Verification items for this drawing (mm, ordinates from the low corner). A direction names the side the tool comes from. Give positions to 0.01 mm unless a question says otherwise; leave off trailing zeros. Loops run counter-clockwise (first coordinate to the right, second up) from the corner with the lowest first, then second, coordinate; pieces in that order, holes last. Notation, with made-up numbers: M -3.75,80 L 17.25,80 A11 ccw 17.25,88 Z; hole C -6.75,12.5 d9. An arc over 180 degrees is marked long. Use a Markdown table: item, result.
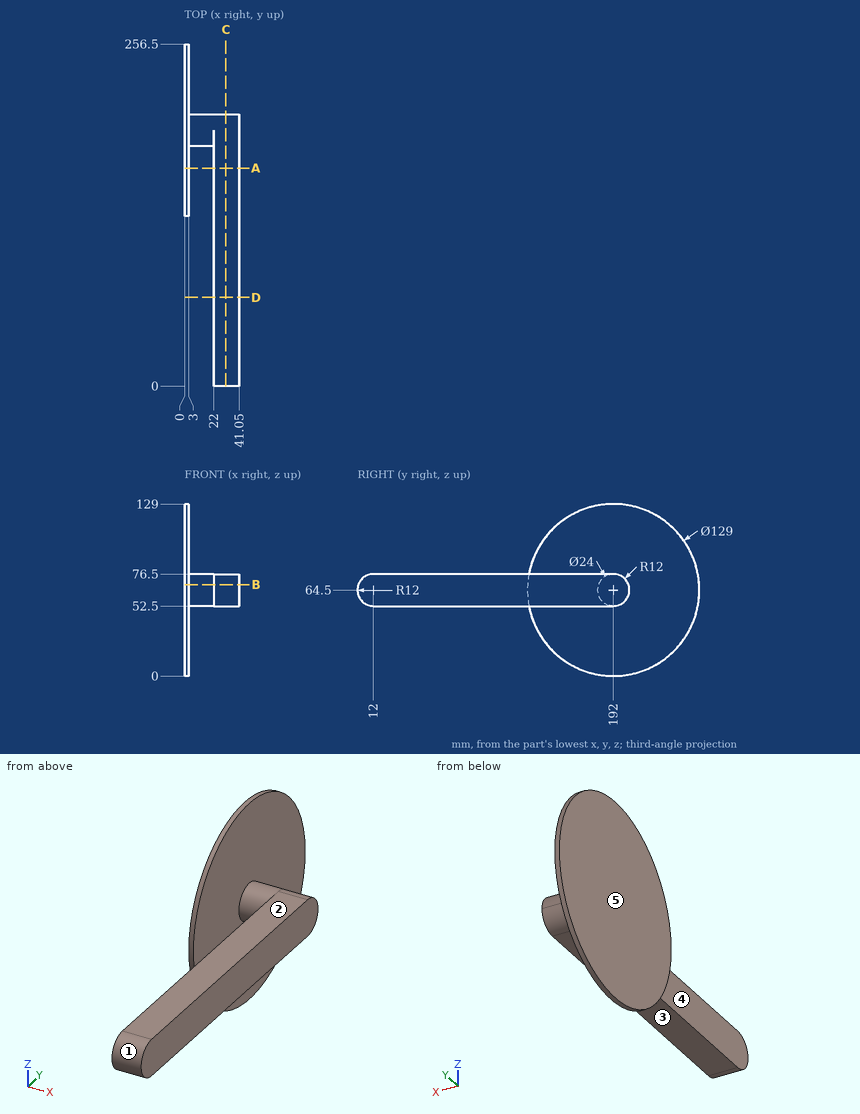
(1) Cross-section at B-B on z = 68.5. Record the cut outline in (x, y), then the cut area to 3 significant figures.
Results below:
| item | result |
|---|---|
| outline | M 0,127.62 L 3,127.62 L 3,180.69 L 22,180.69 L 22,0.69 L 41.05,0.69 L 41.05,203.31 L 3,203.31 L 3,256.38 L 0,256.38 Z |
| area | 4,680 mm^2 |
(2) Cross-section at A-A on y = 163.5. Record the cut outline in (x, z).
Results below:
| item | result |
|---|---|
| outline | M 0,6.64 L 3,6.64 L 3,122.36 L 0,122.36 Z; M 22,52.5 L 41.05,52.5 L 41.05,76.5 L 22,76.5 Z |
(3) Set-up check for the marked faces 1 and 2: record each of +Z, -Z, +X, -X, +Y, -Y from which the full face is reachable in a straight line by a thin tool's end or side.
Results below:
| item | result |
|---|---|
| face 1 | +X, -X, -Y |
| face 2 | +Z, +X, +Y, -Y |
(4) Gauge pin test, flat ends, axial feed: P1, Ø4, axis at x = 29, y = 111.5, coming from the +Z side; P2, Ø15, axis at x = 27, y = 59, coming from the -Z side; P3, Ø12, axis at x = 6.5, z = 14, coming from the -Y side. Record the tip position at first contact, or that the pin passes through.
Results below:
| item | result |
|---|---|
| P1 | z = 76.5 |
| P2 | z = 52.5 |
| P3 | y = 146.41 |
(5) Cross-section at C-C on x = 31. Record the cut outline in (y, z).
Results below:
| item | result |
|---|---|
| outline | M 12,52.5 L 192,52.5 A12 ccw 204,64.5 A12 ccw 192,76.5 L 12,76.5 A12 ccw Z |
(6) Draft check along X on the marked faces 3, 4 and 5. Enter one of: +X half, -X half, draft (parallel to the pull), parting line (faces both ways), or undercut.
Results below:
| item | result |
|---|---|
| face 3 | draft |
| face 4 | undercut |
| face 5 | -X half |
(7) Material ranges on line 1 (X direction, y = 178, z = 64); line 2 (Z direction, x = 29.5, y = 53); line 3 (X direction, y = 188.5, z = 36.5), recorded low to high.
Results below:
| item | result |
|---|---|
| line 1 | 0 to 3, 22 to 41.05 |
| line 2 | 52.5 to 76.5 |
| line 3 | 0 to 3 |
(8) Cross-section at D-D on y = 66.5. Record the cut outline in (x, z), then the cut area to 3 significant figures.
Results below:
| item | result |
|---|---|
| outline | M 22,52.5 L 41.05,52.5 L 41.05,76.5 L 22,76.5 Z |
| area | 457 mm^2 |
